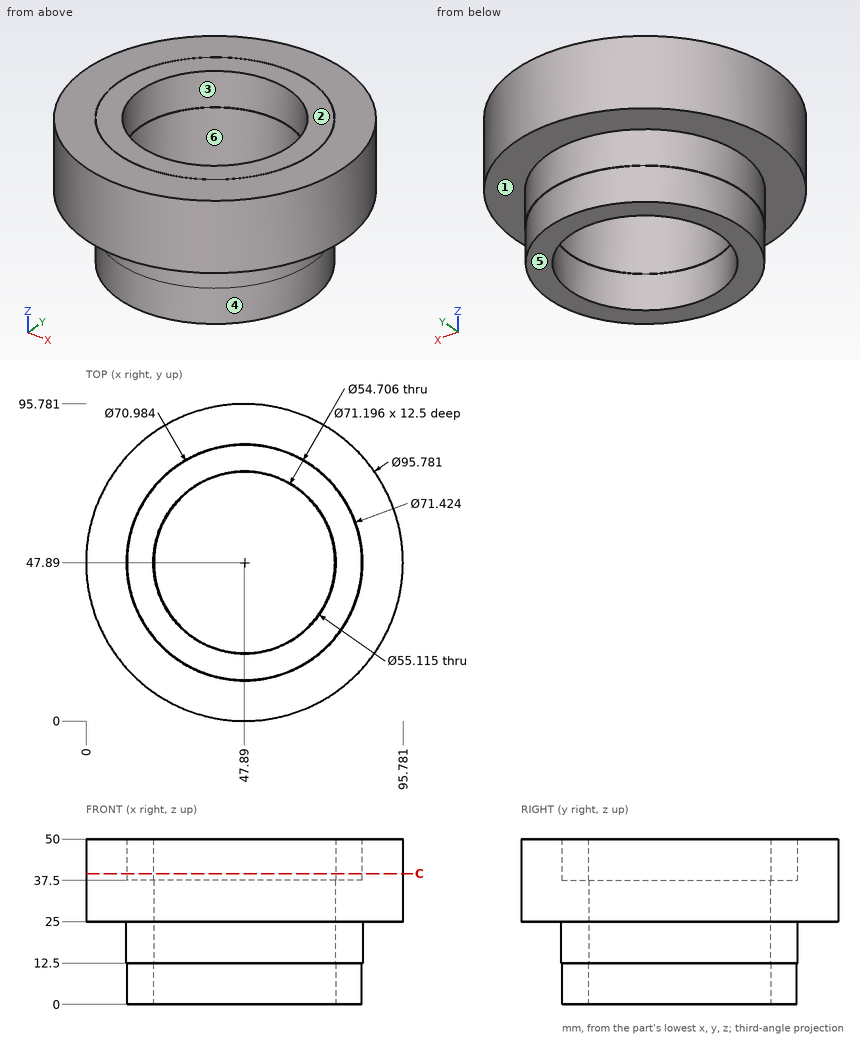
For this review, use the dimensioned drawing (mm, ordinates from the lowest corner) and the shaded views. A direction names the side the tool comes from. Coordinates: 2 decimals unless noted, no trailing zeros. Order: outer loops, then holes, each group sorted by start corner. A loop starts at its lowest first (then second) coordinate and runs counter-clockwise, first axis right, second up. Notation, with made-up numbers: (66, -40) - (115, -40) arc R12 ccw to (115, -24) - close; hole circle Ø3 at (59, 53.25). An arc over 180 degrees is marked (long way). Use one line per item in the form item = value.
Q1. For the marked faces 1, 2 and 3, list the 3-axis set-ups (+Z, -Z, +X, -X, +Y, -Y) from which the entire face can be reached by the end or side of a thin tool; tool diameter is ignored.
Checked values:
face_1 = -Z
face_2 = +Z, +X, -X, +Y, -Y
face_3 = +Z
Q2. Consider section C-C (z = 39.5). Give the boundary of the cut face in (x, y) (1 decimal).
Checked values:
outline = circle Ø95.8 at (47.9, 47.9); circle Ø71 at (47.9, 47.9); hole circle Ø71.2 at (47.9, 47.9); hole circle Ø55.1 at (47.9, 47.9)
Q3. Draft analysis for pull direction X (two halves, no side actions). For the marked faces 4, 5 and 6, state which applies: +X half, -X half, draft (parallel to the pull), parting line (faces both ways), or undercut.
Checked values:
face_4 = parting line
face_5 = draft
face_6 = undercut
Q4. For P1, Ø5, axis at x = 79.5, y = 48.5, coming from the -Z side; P2, Ø10, axis at x = 66.5, z = 31, coming from the -Y side (1 decimal); P3, Ø2, axis at y = 84.5, z = 40.5, coming from the +X side (1 decimal); P4, Ø12, axis at y = 86, z = 12.5, coming from the -X side, all flat-tipped, find the tip position at first contact; note any pin that passes through.
Checked values:
P1 = 0
P2 = 2
P3 = 79.9
P4 = 32.26
Q5. For probe 1 along Y at (x, z) = (16, 44) (1 decimal); probe 2 along X at (y, z) = (47.5, 26); probe 3 along X at (y, z) = (51.5, 15.5) (1 decimal), list the stretches that pass through material, from the lowest coordinate up. Write a range as from..to.
Checked values:
probe_1 = 12.2..32.1, 32.3..63.5, 63.7..83.6
probe_2 = 0..20.54, 75.24..95.78
probe_3 = 12.4..20.8, 75..83.4
